from build123d import *

# Parameters (mm, degrees)
CHAMFER_SIZE       = 2
SKETCH003_R        = 1.939156
POCKET001_DEPTH    = 49.001
POLARPATTERN_COUNT = 6


with BuildPart() as part:
    # Sketch002 → Revolution (revolve)
    with BuildSketch(Plane.XY):
        Polygon((2, 0), (2, 1), (3.4, 1), (3.4, 7), (7, 7), (7, 3), (4, 0), align=None)
    revolve(axis=Axis((0, 0, 0), (0, 1, 0)))

    # Chamfer
    chamfer_edges = [part.edges().sort_by_distance(p)[0] for p in [
        (-3.4, 7, 0),
    ]]
    chamfer(chamfer_edges, length=CHAMFER_SIZE)

    # Sketch003 (on Face4 of Chamfer) → Pocket001 (cut, through all)
    with BuildSketch(Plane(origin=(0, 7, 0), x_dir=(-1, 0, 0), z_dir=(0, 1, 0))):
        with Locations((0, 7.749273)):
            Circle(SKETCH003_R)
    pocket001 = extrude(amount=-POCKET001_DEPTH, mode=Mode.SUBTRACT)

    # PolarPattern: Pocket001 ×6 about axis
    polarpattern_axis = Axis((0, 7, 0), (0, 1, 0))
    for i in range(1, POLARPATTERN_COUNT):
        add(pocket001.rotate(polarpattern_axis, i * 360 / POLARPATTERN_COUNT), mode=Mode.SUBTRACT)


solid = part.part
The listing builds one solid part. Answer for the finished solid, in the listing's coordinates (mm). A direction names the side the tool comes from. Round coordinates to 2 decimals unless told otherwise and drop trailing zeros. Loops run counter-clockwise (first coordinate to the right, second up) from the corner with the lowest first, then second, coordinate; pieces in that order, holes last. Notation, with made-up numbers: M -9.5,40 L 9.5,40 A7 ccw 9.5,46 Z; hole C 68,56 d10. An arc over 180 degrees is marked long. Write each question's results on one line, items separated by ' | '. Start each with the question number.
1) Determine the mould class of faces 3 (the cylindrical face through (3.52, 4.97, -6.05)), 4 (the flat face through (4, 7, -4)), 5 (the flat face through (0, 1, 2.2)) for opening direction X: pulls with the +X half, pulls with the -X half, needs draft (parallel to the pull), parting line crosses it, or undercut.
2) Find section C-C on y = 6. Write down the section's boundary in (x, z).
3) Find section B-B on z = 0. Write down the section's boundary in (x, y).
4) Straight lines are drawn through the part: probe 1 along Z at (x, y) = (0, 2.3); probe 2 along X at (y, z) = (3.7, 0); probe 3 along X at (y, z) = (6.5, 0). For each, find the intervals that lie inside material, in ascending order.
5) Find section A-A on x = 0. Write down the section's boundary in (y, z), plus the area to 3 significant figures.
6) Find section D-D on y = 0.5. Write down the section's boundary in (x, z).
7) Which of the six approach directions +Z, -Z, +X, -X, +Y, -Y give full straight-line access (tool end or side, diameter ignored) to faces 1 (the cylindrical face through (-3.52, 4.97, 6.05)), 2 (the cylindrical face through (-0.74, 3.03, 3.32))?
8) Each of these flat-tipped pins is pushed along its axis until it touches: pin 1 (2.5 mm diameter, centred on x = 0, z = 0, fed in from -Y); pin 2 (4 mm diameter, centred on y = 5, z = 4.5, fed in from -X); pin 3 (1 mm diameter, centred on x = -3, y = 6.5, fed in from +Z); pin 4 (2 mm diameter, centred on y = 6, z = -5, fed in from -X). Where does it stop, or does it pass through?
Final values:
1) face 3: pulls with the +X half | face 4: needs draft | face 5: undercut
2) outline: M -6.73,-1.94 A1.94 cw -5.04,-4.86 A7 ccw -1.69,-6.79 A1.94 cw 1.69,-6.79 A7 ccw 5.04,-4.86 A1.94 cw 6.73,-1.94 A7 ccw 6.73,1.94 A1.94 cw 5.04,4.86 A7 ccw 1.69,6.79 A1.94 cw -1.69,6.79 A7 ccw -5.04,4.86 A1.94 cw -6.73,1.94 A7 ccw Z; hole C 0,0 d8.8
3) outline: M -7,3 L -4,0 L -2,0 L -2,1 L -3.4,1 L -3.4,5 L -5.4,7 L -7,7 Z; M 2,0 L 4,0 L 7,3 L 7,7 L 5.4,7 L 3.4,5 L 3.4,1 L 2,1 Z
4) probe 1: -5.81 to -3.4, 3.4 to 5.81 | probe 2: -7 to -3.4, 3.4 to 7 | probe 3: -7 to -4.9, 4.9 to 7
5) outline: M 0,-4 L 1.81,-5.81 L 7,-5.81 L 7,-5.4 L 5,-3.4 L 1,-3.4 L 1,-2 L 0,-2 Z; M 0,2 L 1,2 L 1,3.4 L 5,3.4 L 7,5.4 L 7,5.81 L 1.81,5.81 L 0,4 Z | area: 29.3 mm²
6) outline: C 0,0 d9; hole C 0,0 d4
7) face 1: +Z, -X, +Y, -Y | face 2: +Y
8) pin 1: through | pin 2: x = -5.34 | pin 3: z = 6.54 | pin 4: x = -5.04
